```python
from build123d import *

# Parameters (mm, degrees)
SKETCH1_R           = 1.524
BOSS_EXTRUDE1_DEPTH = 12.7
SKETCH3_R           = 2.54
BOSS_EXTRUDE2_DEPTH = 3.81


with BuildPart() as part:
    # Sketch1 → Boss-Extrude1 (new body)
    with BuildSketch(Plane(origin=(0, 0, 0), x_dir=(0, 0, -1), z_dir=(1, 0, 0))):
        Polygon((-21.082, 5.388153673), (-15.693846327, 0), (0, 0), (0, 31.7), (-21.082, 31.7), align=None)
        with Locations((-3.048, 28.194)):
            Circle(SKETCH1_R, mode=Mode.SUBTRACT)
        with BuildLine():
            Line((-7.874, 4.318), (-3.048, 4.318))
            ThreePointArc((-3.048, 4.318), (-1.524, 2.794), (-3.048, 1.27))
            Line((-3.048, 1.27), (-7.874, 1.27))
            ThreePointArc((-7.874, 1.27), (-9.398, 2.794), (-7.874, 4.318))
        make_face(mode=Mode.SUBTRACT)
    extrude(amount=BOSS_EXTRUDE1_DEPTH)

    # Sketch3 → Boss-Extrude2 (add)
    with BuildSketch(Plane(origin=(0, -7.846923164, 7.846923164), x_dir=(1, 0, 0), z_dir=(0, -0.7071067811865464, 0.7071067811865488))):
        with Locations(Location((6.35, 14.907225161, 0), (0, 0, 270))):
            Circle(SKETCH3_R)
    extrude(amount=BOSS_EXTRUDE2_DEPTH)


solid = part.part
```
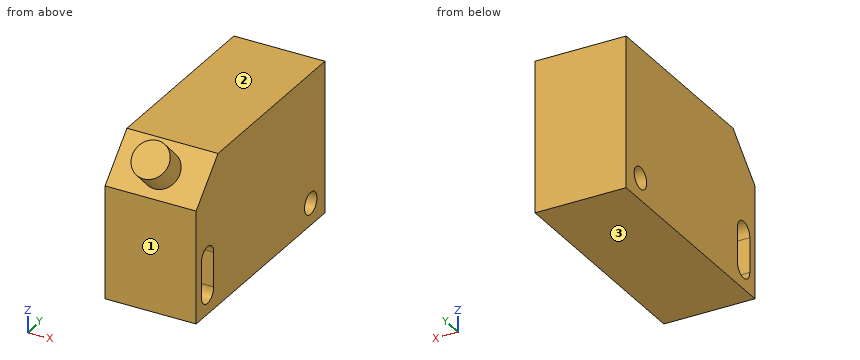
Design review of the part built by this model. Coordinates are the model's own, in mm. Face numbers are marked on the shaded views. A direction names the side the tool comes from. Coordinates: 2 decimals unless noted, no trailing zeros. Order: outer loops, then holes, each group sorted by start corner. A loop starts at its lowest first (then second) coordinate and runs counter-clockwise, first axis right, second up.
1) Take a section at D-D, the plane y = 19. Give the boundary of the cut face in (x, z), and give its area (3 significant figures).
2) Wall thickness on line 1 along Y through (x, z) = (2, 3.75); line 2 along Y through (x, z) = (5.75, 5.75); line 3 along Z through (x, y) = (4, 20.5): over which ranges is each line inside the solid? List them lowest first.
3) For the marked faces 1, 2 and 3, list the 3-axis set-ups (+Z, -Z, +X, -X, +Y, -Y) from which the entire face can be reached by the end or side of a thin tool; tool diameter is ignored.
4) Take a section at C-C, the plane x = 4.5. Give the boundary of the cut face in (y, z), and give its area (3 significant figures).
5) Take a section at A-A, the plane z = 7.25. Give the boundary of the cut face in (x, y), and give its area (3 significant figures).
6) Clearance check with flat-ended pins moving along their axes: pin 1 (1 mm diameter, centred on x = 4, z = 13, fed in from -Y); pin 2 (3 mm diameter, centred on x = 6, y = 8, fed in from +Z); pin 3 (2 mm diameter, centred on y = 2.5, z = 5.5, fed in from +X). State where each tip first meets the part, or that it passes through.
7) Take a section at B-B, the plane z = 2. Give the boundary of the cut face in (x, y), and give its area (3 significant figures).
Returned:
1. outline: (0, 0) - (12.7, 0) - (12.7, 21.08) - (0, 21.08) - close
1. area: 268 mm2
2. line 1: y = 0 to 1.27, 4.32 to 26.84, 29.55 to 31.7
2. line 2: y = 0 to 1.27, 4.32 to 31.7
2. line 3: z = 0 to 21.08
3. face 1: -Z, +X, -X, -Y
3. face 2: +Z, +X, -X, +Y
3. face 3: -Z, +X, -X, +Y, -Y
4. outline: (-1.23, 19.85) - (1.46, 17.16) - (0, 15.69) - (0, 0) - (31.7, 0) - (31.7, 21.08) - (5.39, 21.08) - (3.92, 19.62) - (1.23, 22.31) - close; hole (1.27, 3.05) arc R1.52 ccw to (4.32, 3.05) - (4.32, 7.87) arc R1.52 ccw to (1.27, 7.87) - close; hole circle Ø3.05 at (28.19, 3.05)
4. area: 638 mm2
5. outline: (0, 0) - (12.7, 0) - (12.7, 1.27) - (0, 1.27) - close; (0, 4.32) - (12.7, 4.32) - (12.7, 31.7) - (0, 31.7) - close
5. area: 364 mm2
6. pin 1: stops at y = 0
6. pin 2: stops at z = 21.08
6. pin 3: passes through
7. outline: (0, 0) - (12.7, 0) - (12.7, 1.69) - (0, 1.69) - close; (0, 3.9) - (12.7, 3.9) - (12.7, 27.09) - (0, 27.09) - close; (0, 29.3) - (12.7, 29.3) - (12.7, 31.7) - (0, 31.7) - close
7. area: 346 mm2
